```python
from build123d import *

# Parameters (mm, degrees)
SKETCH1_W           = 6
SKETCH1_H           = 6
BOSS_EXTRUDE1_DEPTH = 5
CUT_EXTRUDE2_DEPTH  = 10
CUT_EXTRUDE3_DEPTH  = 2.5


with BuildPart() as part:
    # Sketch1 → Boss-Extrude1 (new body)
    with BuildSketch(Plane(origin=(0, 0, 0), x_dir=(1, 0, 0), z_dir=(0, 1, 0))):
        Rectangle(SKETCH1_W, SKETCH1_H)
    extrude(amount=BOSS_EXTRUDE1_DEPTH)

    # Sketch5 → Cut-Extrude2 (cut)
    with BuildSketch(Plane.XY.offset(3)):
        with BuildLine():
            Line((-3, 5), (-3, 2.5))
            ThreePointArc((-3, 2.5), (-2.410895752, 4.127135349), (-0.916666667, 5))
            Line((-0.916666667, 5), (-3, 5))
        make_face()
        with BuildLine():
            Line((-3, 0), (-0.916666667, 0))
            ThreePointArc((-0.916666667, 0), (-2.410895752, 0.872864651), (-3, 2.5))
            Line((-3, 2.5), (-3, 0))
        make_face()
    extrude(amount=-CUT_EXTRUDE2_DEPTH, mode=Mode.SUBTRACT)

    # Sketch6 → Cut-Extrude3 (cut)
    with BuildSketch(Plane.XY.offset(3)):
        with BuildLine():
            ThreePointArc((-0.916666667, 5), (-2.410895752, 4.127135349), (-3, 2.5))
            ThreePointArc((-3, 2.5), (-1.589896602, 3.44296939), (-0.916666667, 5))
        make_face()
        with BuildLine():
            Line((0, 0), (-3, 2.5))
            ThreePointArc((-3, 2.5), (-2.410895752, 0.872864651), (-0.916666667, 0))
            Line((-0.916666667, 0), (0, 0))
        make_face()
    extrude(amount=-CUT_EXTRUDE3_DEPTH, mode=Mode.SUBTRACT)


solid = part.part
```
Input: part model. Units: mm. Frame: model coordinates. A direction names the side the tool comes from. Coordinates: 2 decimals unless noted, no trailing zeros. Loops run counter-clockwise (first coordinate to the right, second up) from the corner with the lowest first, then second, coordinate; pieces in that order, holes last.
Q1. Line query: line 1 along Z through (x, y) = (-1.25, 0.3); line 2 along Y through (x, z) = (-1.5, -0.05); line 3 along X through (y, z) = (3.25, -0.85). Output: solid intervals per line, ascending.
Results are:
line 1: z = -3 to 0.5
line 2: y = 0.18 to 4.82
line 3: x = -2.89 to 3
Q2. Contact query for flat-ended pins moving along their axis: pin 1 (1.5 mm diameter, centred on x = -1, z = 1.5, fed in from -Y); pin 2 (1 mm diameter, centred on x = -2, y = 4, fed in from +Z). Output: stop coordinate, or through.
Results are:
pin 1: stops at y = 0.21
pin 2: stops at z = 0.5
Q3. Section B-B, the plane y = 3.55. Return the cut outline in (x, z).
Results are:
outline: (-2.77, -3) - (3, -3) - (3, 3) - (-1.5, 3) - (-1.5, 0.5) - (-2.77, 0.5) - close
Q4. Section A-A, the plane z = 2. Return the cut outline in (x, y).
Results are:
outline: (-3, 2.5) - (0, 0) - (3, 0) - (3, 5) - (-0.92, 5) arc R3 cw to start
Q5. Section D-D, the plane z = -0.95. Return the cut outline in (x, y), and give its area (3 significant figures).
Results are:
outline: (-0.92, 0) - (3, 0) - (3, 5) - (-0.92, 5) arc R2.54 ccw to start
area: 27.4 mm2
Q6. Set-up query: faces 1 (the flat face through (-1.479, 1.233, 1.768)), 2 (the flat face through (1, 2, 3)), 3 (the flat face through (-2, 4, 0.5)). Return all of +Z, -Z, +X, -X, +Y, -Y with unobstructed straight access to the full face (end or side cutting, diameter ignored); none if empty.
Results are:
face 1: +Z, -X, -Y
face 2: +Z, +X, -X, +Y, -Y
face 3: +Z, -X, +Y
Q7. Section C-C, the plane x = -2. Return the cut outline in (y, z), and give its area (3 significant figures).
Results are:
outline: (0.48, -3) - (4.52, -3) - (4.52, 0.5) - (3.04, 0.5) - (3.04, 3) - (1.67, 3) - (1.67, 0.5) - (0.48, 0.5) - close
area: 17.6 mm2
